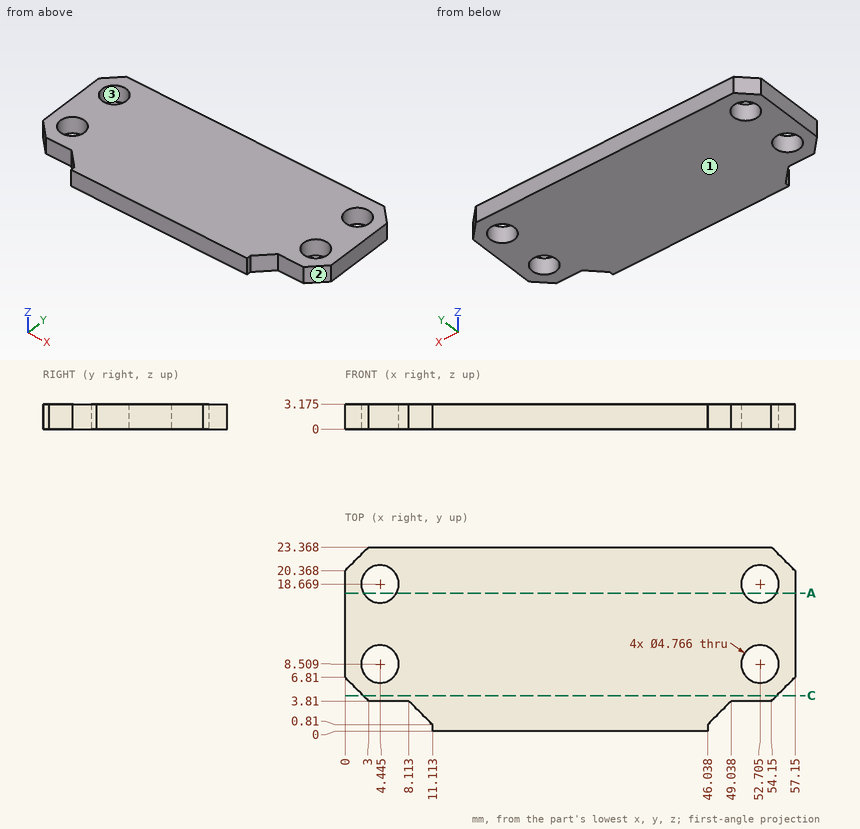
Design review of the part shown in the three views and the two pictorial views. Dimensions are in mm from the part's minimum x, y and z. Round coordinates to 2 decimals unless told otherwise and drop trailing zeros. Order: outer loops, then holes, each group sorted by start corner. A loop starts at its lowest first (then second) coordinate and runs counter-clockwise, first axis right, second up. Notation, with made-up numbers: M 44,1 L 76,1 A15 ccw 76,21 Z; hole C 89,37.5 d10. An arc over 180 degrees is marked long. Put each result on its own line as item: value.
Q1. Draft analysis for pull direction X (two halves, no side actions). For the marked faces 1, 2 and 3, state which applies: released by +X, released by -X, zero draft, split by the parting line, or undercut.
Reported:
face 1: zero draft
face 2: released by +X
face 3: undercut
Q2. Insertion check: pin 1 Ø0.9 at (y, z) = (0.5, 1) entering from -X; pin 2 Ø1 at (x, z) = (52, 2) entering from -Y. Each pin has a flat end and moves straight along its axis. Give the tip position at first contact, or say it passes through.
Reported:
pin 1: x = 10.97
pin 2: y = 3.81
Q3. To check wall thickness, follow line 1 (Y direction, x = 4.5, z = 1.2); line 2 (X direction, y = 19.5, z = 2.25); line 3 (Y direction, x = 8, z = 2.1). State the ranges of each line that lie inside material, in increasing order.
Reported:
line 1: 3.81 to 6.13, 10.89 to 16.29, 21.05 to 23.37
line 2: 0 to 2.21, 6.68 to 50.47, 54.94 to 57.15
line 3: 3.81 to 23.37
Q4. Consider section A-A (y = 17.5). State how many separate pieces and enclosed holes the cut face has, and give its area (3 significant figures).
Reported:
separate pieces: 3
enclosed holes: 0
area: 155 mm²
Q5. Consider section C-C (y = 4.5). State the section outline as (x, z) points (1 decimal), and give its area (3 significant figures).
Reported:
outline: M 2.3,0 L 54.8,0 L 54.8,3.2 L 2.3,3.2 Z
area: 167 mm²
